Work out the finished part from the listing and answer in its coordinate system (mm). A direction names the side the tool comes from. Give positions to 0.01 mm unless a question says otherwise; leave off trailing zeros. Loops run counter-clockwise (first coordinate to the right, second up) from the corner with the lowest first, then second, coordinate; pieces in that order, holes last. Notation, with made-up numbers: (-3, -38) -> (16, -38) arc R20 ccw to (16, -34) -> close; hole circle Ø8 at (-30, -28.5). An arc over 180 degrees is marked (long way). Answer as CSV lines item,"result". Start each with the question number.
1. Find section D-D, the plane y = 5.5. Count the separate pieces of the cut face and the enclosed holes in it, and give its area (3 significant figures).
2. Find the intervals of material crossed by line 1 along Z through (x, y) = (19.5, 53.25); line 2 along X through (y, z) = (48, 28) (3 decimals); line 3 along X through (y, z) = (50, -3.5), in increasing order.
3. Find section A-A, the plane z = 11.5. Give the vertices of the cut face in (x, y), and give its area (3 significant figures).
4. Find section C-C, the plane z = 25. Give the vertices of the cut face in (x, y) (3 decimals).
5. A tool of negligible diameter and unlimited length cuts with its end or side. For faces 1 (the face through (19.574, 13.408, 28.282)), 2 (the face through (-23, 22, -6.5)), 3 (the face through (-22, 44, 24)), from which of +Z, -Z, +X, -X, +Y, -Y can it reach the whole face along a straight path? Write none if from no direction.
6. Determine the mould class of faces 4 (the face through (-24, 29, -11)), 5 (the face through (0, 16, 30.08)), 6 (the face through (0, 46, -6.5)) for opening direction Z: +Z half, -Z half, draft (parallel to the pull), parting line (faces both ways), or undercut.
7. Find section B-B, the plane y = 27.5. Give the vertices of the cut face in (x, z).
8. Flat-ended cylindrical pins translate along their axes: pin 1 Ø12 at (y, z) = (11, 10) entering from -X; pin 2 Ø2.5 at (x, y) = (11, 46.5) entering from -Z; pin 3 Ø1.5 at (x, z) = (2.5, -11) entering from +Y. Find the tip coordinate at first contact, or state that the pin passes through.
Autodesk Inventor part; units mm, degrees
ref_plane "YZ Plane" through (0, 0, 0) normal (1, 0, 0) x (0, 1, 0)
ref_plane "XZ Plane" through (0, 0, 0) normal (0, 1, 0) x (-1, 0, 0)
ref_plane "XY Plane" through (0, 0, 0) normal (0, 0, 1) x (1, 0, 0)
sketch "Sketch1" plane through (0, 0, 0) normal (0, 1, 0) x (-1, 0, 0)
  line L0 (101.6, 101.6) -> (-101.6, 101.6)
  line L1 (-101.6, 101.6) -> (-101.6, -101.6)
  line L2 (-101.6, -101.6) -> (101.6, -101.6)
  line L3 (101.6, -101.6) -> (101.6, 101.6)
  circle A0 centre (0, 0) radius 2.5
  line L4 (9.525, -6.5) -> (-9.525, -6.5)
  line L5 (0, 0) -> (0, 8)
  line L6 (-14.5, -6.5) -> (-14.5, 22.5)
  line L7 (14.5, 22.5) -> (14.5, -6.5)
  circle A1 centre (0, 8) radius 14
  line L8 (-14.5, 22.5) -> (14.5, 22.5)
  line L9 (14.5, -6.5) -> (-14.5, -6.5)
  line L10 (-24.5, 32.5) -> (24.5, 32.5)
  line L11 (24.5, 32.5) -> (24.5, -16.5)
  line L12 (24.5, -16.5) -> (-24.5, -16.5)
  line L13 (-24.5, -16.5) -> (-24.5, 32.5)
  line L14 (-9.525, 22.5) -> (9.525, 22.5)
  line L15 (9.525, 22.5) -> (9.525, 27.58)
  line L16 (9.525, 27.58) -> (-9.525, 27.58)
  line L17 (-9.525, 27.58) -> (-9.525, 22.5)
  point P0 (9.525, 22.5)
  point P1 (-9.525, -6.5)
  dimension "d0" = 203.2
  dimension "d1" = 203.2
  dimension "d2" = 8
  dimension "d3" = 28
  dimension "d4" = 29
  dimension "d5" = 29
  dimension "d6" = 14.5
  dimension "d7" = 10
  dimension "d8" = 10
  dimension "d9" = 10
  dimension "d10" = 10
  dimension "d11" = 5.08
  dimension "d12" = 9.525
  dimension "d13" = 9.525
  dimension "d14" = 101.6
  dimension "d15" = 101.6
extrude "Extrusion1" add sketch "Sketch1" along normal blind 56.5 contours A0 | L4 L9 L6 L8 L7 | L8 L17 L16 L15 | A1 | L10 L11 L12 L13
sketch "Sketch2" plane through (0, 56.5, 0) normal (0, 1, 0) x (1, 0, 0)
  line L0 (101.6, 101.6) -> (-101.6, 101.6)
  line L1 (-101.6, 101.6) -> (-101.6, -101.6)
  line L2 (-101.6, -101.6) -> (101.6, -101.6)
  line L3 (101.6, -101.6) -> (101.6, 101.6)
  circle A0 centre (0, 0) radius 2.5
  line L4 (-9.525, 6.5) -> (9.525, 6.5)
  line L5 (0, 0) -> (0, -8)
  line L6 (14.5, 6.5) -> (14.5, -22.5)
  line L7 (-14.5, -22.5) -> (-14.5, 6.5)
  circle A1 centre (0, -8) radius 14
  line L8 (14.5, -22.5) -> (-14.5, -22.5)
  line L9 (-14.5, 6.5) -> (14.5, 6.5)
  line L10 (24.5, -32.5) -> (-24.5, -32.5)
  line L11 (-24.5, -32.5) -> (-24.5, 16.5)
  line L12 (-24.5, 16.5) -> (24.5, 16.5)
  line L13 (24.5, 16.5) -> (24.5, -32.5)
  line L14 (9.525, -22.5) -> (-9.525, -22.5)
  line L15 (-9.525, -22.5) -> (-9.525, -27.58)
  line L16 (-9.525, -27.58) -> (9.525, -27.58)
  line L17 (9.525, -27.58) -> (9.525, -22.5)
  point P0 (9.525, 22.5)
  point P1 (-9.525, -6.5)
  dimension "d18" = 203.2
  dimension "d19" = 203.2
  dimension "d20" = 8
  dimension "d21" = 28
  dimension "d22" = 29
  dimension "d23" = 29
  dimension "d24" = 14.5
  dimension "d25" = 10
  dimension "d26" = 10
  dimension "d27" = 10
  dimension "d28" = 10
  dimension "d29" = 5.08
  dimension "d30" = 9.525
  dimension "d31" = 9.525
  dimension "d32" = 101.6
  dimension "d33" = 101.6
extrude "Extrusion2" cut sketch "Sketch2" against normal blind 19.5 contours A0 | L4 L9 L6 L8 L7 | L8 L17 L16 L15 | A1
sketch "Sketch4" plane through (0, 56.5, 0) normal (0, 1, 0) x (1, 0, 0)
  circle A0 centre (-17.508, -8) radius 2
  circle A1 centre (17.4854, -8) radius 2
  circle A2 centre (17.4854, -8) radius 2
  circle A3 centre (0, -8.01) radius 14
  circle A4 centre (0, -0.01) radius 2.5
  circle A5 centre (-19.4934, 12.0285) radius 2.2448
  circle A6 centre (19.5, 12.0285) radius 2.3104
  circle A7 centre (19.5, -28.5182) radius 2.2008
  circle A8 centre (-19.4934, -28.5182) radius 2.3894
  point P0 (0, 0)
  dimension "d37" = 34.9934
  dimension "d38" = 28
  dimension "d39" = 8
  dimension "d65" = 8
  dimension "d66" = 8
hole "Hole1" at (-17.508, 56.5, 8) at (17.4854, 56.5, 8) at (-19.4934, 56.5, 28.5182) at (19.5, 56.5, 28.5182) at (-19.4934, 56.5, -12.0285) at (19.5, 56.5, -12.0285) direction (0, -1, 0) diameter 2.85 depth 12.7 tip angle 118 countersink diameter 3.0226 countersink angle 82
sketch "Sketch5" plane through (0, 0, 0) normal (0, -1, 0) x (1, 0, 0)
  circle A0 centre (-19.4934, 28.5182) radius 1.425
  circle A1 centre (-19.4934, 28.5182) radius 1.425
  circle A2 centre (19.5, 28.5182) radius 1.425
  circle A3 centre (19.5, 28.5182) radius 1.425
  circle A4 centre (19.5, -12.0285) radius 1.425
  circle A5 centre (19.5, -12.0285) radius 1.425
  circle A6 centre (-19.4934, -12.0285) radius 1.5113
  circle A7 centre (-19.4934, -12.0285) radius 1.5113
  point P0 (0, 0)
hole "Hole2" at (19.5, 0, -12.0285) at (-19.4934, 0, -12.0285) at (-19.4934, 0, 28.5182) at (19.5, 0, 28.5182) direction (0, 1, 0) diameter 2.85 depth 12.7 tip angle 118 countersink diameter 3.0226 countersink angle 82
sketch "Sketch6" plane through (-24.5, 0, 32.5) normal (0, 0, 1) x (1, 0, 0)
  line L0 (34.025, 56.5) -> (34.025, 37)
  line L1 (14.975, 56.5) -> (34.025, 56.5)
  line L2 (34.025, 56.5) -> (34.025, 46.75)
  line L3 (34.025, 46.75) -> (14.975, 46.75)
  line L4 (14.975, 46.75) -> (14.975, 56.5)
  point P0 (24.5, 0)
extrude "Extrusion3" cut sketch "Sketch6" against normal blind 25.4
sketch "Sketch8" plane through (0, 56.5, 0) normal (0, 1, 0) x (1, 0, 0)
  line L0 (-24.5, -3) -> (24.5, -3)
  line L1 (24.5, -3) -> (24.5, -13)
  line L2 (24.5, -13) -> (-24.5, -13)
  line L3 (-24.5, -13) -> (-24.5, -3)
  line L4 (14.5, 6.5) -> (14.5, -22.5)
  line L5 (14.5, -3) -> (14.5, -13)
  line L6 (-14.5, -22.5) -> (-14.5, 6.5)
  line L7 (-14.5, -3) -> (-14.5, -13)
  line L8 (24.5, -32.5) -> (24.5, 16.5)
  line L9 (-24.5, 16.5) -> (-24.5, -32.5)
  point P0 (0, 0)
  dimension "d58" = 10
  dimension "d60" = 0
  dimension "d61" = 0
  dimension "d62" = 3
extrude "Extrusion4" cut sketch "Sketch8" against normal blind 2 contours L0 L6 L2 L3 | L0 L1 L2 L4
sketch "Sketch9" plane through (0, 56.5, 0) normal (0, 1, 0) x (1, 0, 0)
  line L0 (-14.5, 6.5) -> (14.5, 6.5)
  line L1 (24.5, 16.5) -> (-24.5, 16.5)
  line L2 (-14.5, 6.5) -> (14.5, 6.5)
  line L3 (14.5, 6.5) -> (14.5, 16.5)
  line L4 (14.5, 16.5) -> (-14.5, 16.5)
  line L5 (-14.5, 16.5) -> (-14.5, 6.5)
  line L6 (14.5, 6.5) -> (14.5, -3)
  line L7 (-14.5, 11.5) -> (14.5, 11.5)
  line L8 (-24.5, 16.5) -> (-24.5, -32.5)
  line L9 (-14.5, 6.5) -> (-24.5, 6.5)
  line L10 (-24.5, 6.5) -> (-24.5, -22.5)
  line L11 (-24.5, -22.5) -> (-14.5, -22.5)
  line L12 (-14.5, -22.5) -> (-14.5, 6.5)
  line L13 (-9.525, -22.5) -> (-14.5, -22.5)
  line L14 (-20.5, 6.5) -> (-20.5, -22.5)
  line L15 (24.5, -32.5) -> (24.5, 16.5)
  line L16 (24.5, -22.5) -> (20.5, -22.5)
  line L17 (20.5, -22.5) -> (20.5, 6.5)
  line L18 (20.5, 6.5) -> (24.5, 6.5)
  line L19 (24.5, 6.5) -> (24.5, -22.5)
  line L20 (-24.5, -32.5) -> (24.5, -32.5)
  line L21 (14.5, -32.5) -> (14.5, -30.08)
  line L22 (14.5, -30.08) -> (-14.5, -30.08)
  line L23 (-14.5, -30.08) -> (-14.5, -32.5)
  line L24 (-9.525, -27.58) -> (9.525, -27.58)
  point P0 (0, 0)
  point P1 (-14.5, 16.5)
  dimension "d67" = 0
  dimension "d68" = 5
  dimension "d69" = 0
  dimension "d71" = 4
  dimension "d72" = 4
  dimension "d98" = 2.5
extrude "Extrusion5" cut sketch "Sketch9" against normal through all contours L5 L1 L3 L7 | L14 L11 L8 L9 | L15 L16 L17 L18 | L23 L22 L21 L20
sketch "Sketch11" plane through (0, 37, 0) normal (0, 1, 0) x (1, 0, 0)
  line L0 (-20.5, -3) -> (-14.5, -3)
  line L1 (20.5, -13) -> (20.5, -3)
  line L2 (-20.5, -3) -> (20.5, -3)
  line L3 (20.5, -3) -> (20.5, -13)
  line L4 (20.5, -13) -> (-20.5, -13)
  line L5 (-20.5, -13) -> (-20.5, -3)
  point P0 (0, 0)
  dimension "d75" = 41
  dimension "d76" = 10
sketch "Sketch12" plane through (14.5, 56.5, -11.5) normal (0, 0, -1) x (-1, 0, 0)
  line L0 (0, 0) -> (-6, 0)
  line L1 (29, 0) -> (29, -19.5)
  line L2 (0, 0) -> (29, 0)
  line L3 (29, 0) -> (29, -2)
  line L4 (29, -2) -> (0, -2)
  line L5 (0, -2) -> (0, 0)
  point P0 (14.5, -56.5)
  dimension "d77" = 2
extrude "Extrusion6" cut sketch "Sketch12" against normal blind 25.4
sketch "Sketch13" plane through (0, 37, 0) normal (0, 1, 0) x (1, 0, 0)
  line L0 (0, 0) -> (7.62, 0)
  line L1 (7.62, 0) -> (7.62, -15.24)
  line L2 (7.62, -15.24) -> (0, -15.24)
  line L3 (0, -15.24) -> (0, 0)
  line L4 (0, 0) -> (-7.62, 0)
  line L5 (-7.62, 0) -> (-7.62, -15.24)
  line L6 (-7.62, -15.24) -> (0, -15.24)
  line L7 (0, -15.24) -> (0, 0)
  line L8 (14.5, 6.5) -> (-14.5, 6.5)
  line L9 (-9.525, -27.58) -> (9.525, -27.58)
  dimension "d80" = 7.62
  dimension "d81" = 15.24
  dimension "d82" = 7.62
  dimension "d86" = 15.24
extrude "Extrusion7" cut sketch "Sketch13" against normal through all
sketch "Sketch14" plane through (0, 56.5, 0) normal (0, 1, 0) x (1, 0, 0)
  line L0 (-14.5, 16.5) -> (-24.5, 16.5)
  line L1 (24.5, 6.5) -> (24.5, 16.5)
  line L2 (-24.5, 16.5) -> (24.5, 16.5)
  line L3 (24.5, 16.5) -> (24.5, 16)
  line L4 (24.5, 16) -> (-24.5, 16)
  line L5 (-24.5, 16) -> (-24.5, 16.5)
  line L6 (24.5, 16.5) -> (14.5, 16.5)
  line L7 (9.525, -32.5) -> (24.5, -32.5)
  line L8 (24.5, 16.5) -> (24, 16.5)
  line L9 (24, 16.5) -> (24, -32.5)
  line L10 (24, -32.5) -> (24.5, -32.5)
  line L11 (24.5, -32.5) -> (24.5, 16.5)
  line L12 (-24.5, -22.5) -> (-24.5, -32.5)
  line L13 (24.5, -32.5) -> (-24.5, -32.5)
  line L14 (-24.5, -32.5) -> (-24.5, -32)
  line L15 (-24.5, -32) -> (24.5, -32)
  line L16 (24.5, -32) -> (24.5, -32.5)
  line L17 (-24.5, -32.5) -> (-9.525, -32.5)
  line L18 (-24.5, -32.5) -> (-24, -32.5)
  line L19 (-24, -32.5) -> (-24, 16.5)
  line L20 (-24, 16.5) -> (-24.5, 16.5)
  line L21 (-24.5, 16.5) -> (-24.5, -32.5)
  point P0 (0, 0)
  point P1 (-24.5, 16)
  point P2 (24, 16)
  point P3 (24, -32)
  point P4 (-24, -32)
  point P5 (-24, 16)
  dimension "d89" = 0.5
  dimension "d90" = 0.5
  dimension "d91" = 0.5
  dimension "d92" = 0.5
extrude "Extrusion8" cut sketch "Sketch14" against normal through all contours L2 L9 L4 L19 L0 | L19 L4 L5 L0 | L19 L15 L12 L21 L4 | L2 L1 L4 L9 | L4 L1 L11 L15 L9 | L19 L13 L12 L15 | L15 L9 L7 L13 L19 | L15 L11 L7 L9
sketch "Sketch18" plane through (0, 56.5, 0) normal (0, 1, 0) x (1, 0, 0)
  line L0 (-20.5, -22.5) -> (-20.5, 6.5)
  line L1 (-24, -22.5) -> (-20.5, -22.5)
  line L2 (-20.5, 6.5) -> (-22.5, 6.5)
  line L3 (-22.5, 6.5) -> (-22.5, -22.5)
  line L4 (-22.5, -22.5) -> (-20.5, -22.5)
  line L5 (-20.5, -22.5) -> (-20.5, 6.5)
  line L6 (-20.5, 6.5) -> (-22.5, 6.5)
  line L7 (-22.5, 6.5) -> (-22.5, 8)
  line L8 (-22.5, 8) -> (-20.5, 8)
  line L9 (-20.5, 8) -> (-20.5, 6.5)
  line L10 (-20.5, -22.5) -> (-22.5, -22.5)
  line L11 (-22.5, -22.5) -> (-22.5, -24)
  line L12 (-22.5, -24) -> (-20.5, -24)
  line L13 (-20.5, -24) -> (-20.5, -22.5)
  line L14 (-14.5, 16) -> (-14.5, 11.5)
  line L15 (14.5, 16) -> (14.5, -3)
  line L16 (-14.5, 11.5) -> (14.5, 11.5)
  line L17 (14.5, 11.5) -> (14.5, 13.5)
  line L18 (14.5, 13.5) -> (-14.5, 13.5)
  line L19 (-14.5, 13.5) -> (-14.5, 11.5)
  line L20 (14.5, 13.5) -> (16, 13.5)
  line L21 (16, 13.5) -> (16, 11.5)
  line L22 (16, 11.5) -> (14.5, 11.5)
  line L23 (14.5, 11.5) -> (14.5, 13.5)
  line L24 (-14.5, 13.5) -> (-16, 13.5)
  line L25 (-16, 13.5) -> (-16, 11.5)
  line L26 (-16, 11.5) -> (-14.5, 11.5)
  line L27 (-14.5, 11.5) -> (-14.5, 13.5)
  line L28 (20.5, -3) -> (20.5, 6.5)
  line L29 (20.5, -22.5) -> (24, -22.5)
  line L30 (20.5, 6.5) -> (22.5, 6.5)
  line L31 (22.5, 6.5) -> (22.5, -22.5)
  line L32 (22.5, -22.5) -> (20.5, -22.5)
  line L33 (20.5, -22.5) -> (20.5, 6.5)
  line L34 (20.5, 6.5) -> (22.5, 6.5)
  line L35 (22.5, 6.5) -> (22.5, 8)
  line L36 (22.5, 8) -> (20.5, 8)
  line L37 (20.5, 8) -> (20.5, 6.5)
  line L38 (20.5, -22.5) -> (22.5, -22.5)
  line L39 (22.5, -22.5) -> (22.5, -24)
  line L40 (22.5, -24) -> (20.5, -24)
  line L41 (20.5, -24) -> (20.5, -22.5)
  line L42 (-14.5, -30.08) -> (14.5, -30.08)
  line L43 (14.5, -30.08) -> (14.5, -28.08)
  line L44 (14.5, -28.08) -> (-14.5, -28.08)
  line L45 (-14.5, -28.08) -> (-14.5, -30.08)
  line L46 (14.5, -28.08) -> (16, -28.08)
  line L47 (16, -28.08) -> (16, -30.08)
  line L48 (16, -30.08) -> (14.5, -30.08)
  line L49 (14.5, -30.08) -> (14.5, -28.08)
  line L50 (-14.5, -28.08) -> (-16, -28.08)
  line L51 (-16, -28.08) -> (-16, -30.08)
  line L52 (-16, -30.08) -> (-14.5, -30.08)
  line L53 (-14.5, -30.08) -> (-14.5, -28.08)
  point P0 (0, 0)
  point P1 (14.5, 11.5)
  dimension "d99" = 2
  dimension "d100" = 1.5
  dimension "d101" = 2
  dimension "d102" = 2
  dimension "d103" = 1.5
  dimension "d104" = 1.5
  dimension "d105" = 2
  dimension "d106" = 1.5
  dimension "d107" = 1.5
  dimension "d108" = 2
  dimension "d109" = 1.5
  dimension "d110" = 1.5
  dimension "d115" = 1.5
extrude "Extrusion9" cut sketch "Sketch18" against normal blind 25.4
sketch "Sketch19" plane through (-16, 56.5, 28.08) normal (0, 0, 1) x (1, 0, 0)
  line L0 (6.475, -9.75) -> (25.525, -9.75)
  line L1 (1.5, -19.5) -> (30.5, -19.5)
  line L2 (6.475, -9.75) -> (26.0764, -9.75)
  line L3 (26.0764, -9.75) -> (26.0764, -19.5)
  line L4 (26.0764, -19.5) -> (6.475, -19.5)
  line L5 (6.475, -19.5) -> (6.475, -9.75)
  point P0 (16, -56.5)
  point P1 (6.475, -19.5)
extrude "Extrusion10" cut sketch "Sketch19" against normal blind 25.4
sketch "Sketch20" plane through (20.5, 54.5, 3) normal (1, 0, 0) x (0, 0, -1)
  point P0 (3, -54.5)
equation "\"d86\" = d81"
equation "\"d100\" = d115"
equation "\"d103\" = d115"
equation "\"d104\" = d115"
equation "\"d106\" = d115"
equation "\"d107\" = d115"
equation "\"d109\" = d115"
equation "\"d110\" = d115"
properties part number "Motor_Holder"
Resolved:
1,separate pieces,"1"
1,enclosed holes,"5"
1,area,"1,660 mm^2"
2,line 1,"z = -16 to -13.45, -10.6 to 27.09, 29.94 to 32"
2,line 2,"x = -24 to -20.821, -18.166 to -9.525, 9.525 to 18.173, 20.827 to 24"
2,line 3,"x = -20.5 to -14.5, 14.5 to 20.5"
3,outline,"(-20.5, 0) -> (-7.62, 0) -> (-7.62, 37) -> (-14.5, 37) -> (-14.5, 54.5) -> (-20.5, 54.5) -> close; (7.62, 0) -> (20.5, 0) -> (20.5, 54.5) -> (14.5, 54.5) -> (14.5, 37) -> (7.62, 37) -> close"
3,area,"1,160 mm^2"
4,outline,"(-24, 0) -> (24, 0) -> (24, 56.5) -> (9.525, 56.5) -> (9.525, 46.75) -> (10.076, 46.75) -> (10.076, 37) -> (-9.525, 37) -> (-9.525, 56.5) -> (-24, 56.5) -> close"
5,face 1,"-Y"
5,face 2,"-X, +Y, -Y"
5,face 3,"+Y"
6,face 4,"draft"
6,face 5,"+Z half"
6,face 6,"undercut"
7,outline,"(-24, -16) -> (-14.5, -16) -> (-14.5, -11.5) -> (14.5, -11.5) -> (14.5, -16) -> (24, -16) -> (24, -6.5) -> (20.5, -6.5) -> (20.5, 22.5) -> (24, 22.5) -> (24, 32) -> (14.5, 32) -> (14.5, 30.08) -> (-14.5, 30.08) -> (-14.5, 32) -> (-24, 32) -> (-24, 22.5) -> (-20.5, 22.5) -> (-20.5, -6.5) -> (-24, -6.5) -> close; hole (-7.62, 0) -> (7.62, 0) -> (7.62, 15.24) -> (-7.62, 15.24) -> close"
8,pin 1,"stops at x = -20.5"
8,pin 2,"stops at z = -11.5"
8,pin 3,"stops at y = 54.5"
